The drawing under review shows one solid part. Ordinate dimensions are in mm from its lowest x, y, z. Coordinates: 2 decimals unless noted, no trailing zeros. Loops run counter-clockwise (first coordinate to the right, second up) from the corner with the lowest first, then second, coordinate; pieces in that order, holes last.
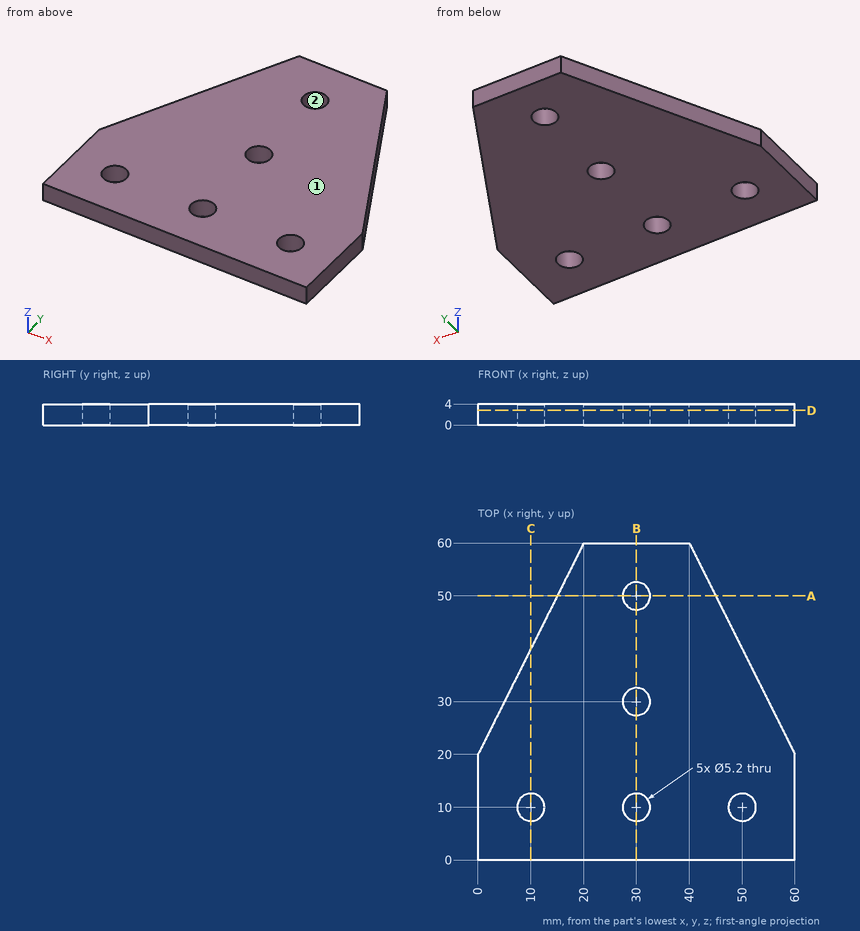
Q1. Take a section at C-C, the plane x = 10. Write out the cut boundary in (y, z), then the cut area to 3 significant figures.
Q2. Clearance check with a flat-ended pin moving along its axis: pin 1 Ø3 at (x, y) = (10, 10) entering from -Z (1 decimal). State where the tip first meets the part, or that it passes through.
Q3. Take a section at A-A, the plane y = 50. Write out the cut boundary in (x, z).
Q4. For line 1 (Y direction, x = 30, z = 2.4); line 2 (Y direction, x = 10, z = 2.55); line 3 (X direction, y = 8, z = 2.6), list the stretches that pass through material, from the lowest coordinate up.
Q5. Take a section at D-D, the plane z = 2.8. Write out the cut boundary in (x, y), then the cut area to 3 significant figures.
Q6. The part is to be moulded in two halves that separate along X. For the marked faces 1 and 2, say which applies: pulls with the +X half, pulls with the -X half, needs draft (parallel to the pull), parting line crosses it, or undercut.
Q7. Take a section at B-B, the plane x = 30. Write out the cut boundary in (y, z), then the cut area to 3 significant figures.
Entries:
1. outline: (0, 0) - (7.4, 0) - (7.4, 4) - (0, 4) - close; (12.6, 0) - (40, 0) - (40, 4) - (12.6, 4) - close
1. area: 139 mm2
2. pin 1: passes through
3. outline: (15, 0) - (27.4, 0) - (27.4, 4) - (15, 4) - close; (32.6, 0) - (45, 0) - (45, 4) - (32.6, 4) - close
4. line 1: y = 0 to 7.4, 12.6 to 27.4, 32.6 to 47.4, 52.6 to 60
4. line 2: y = 0 to 7.4, 12.6 to 40
4. line 3: x = 0 to 8.34, 11.66 to 28.34, 31.66 to 48.34, 51.66 to 60
5. outline: (0, 0) - (60, 0) - (60, 20) - (40, 60) - (20, 60) - (0, 20) - close; hole circle Ø5.2 at (10, 10); hole circle Ø5.2 at (30, 10); hole circle Ø5.2 at (30, 30); hole circle Ø5.2 at (30, 50); hole circle Ø5.2 at (50, 10)
5. area: 2,690 mm2
6. face 1: needs draft
6. face 2: undercut
7. outline: (0, 0) - (7.4, 0) - (7.4, 4) - (0, 4) - close; (12.6, 0) - (27.4, 0) - (27.4, 4) - (12.6, 4) - close; (32.6, 0) - (47.4, 0) - (47.4, 4) - (32.6, 4) - close; (52.6, 0) - (60, 0) - (60, 4) - (52.6, 4) - close
7. area: 178 mm2
